from build123d import *

# Parameters (mm, degrees)
SWEEP_THIN1_PROFILE_R   = 10
SWEEP_THIN1_PROFILE_R_2 = 7
CUT_EXTRUDE1_DEPTH      = 533.134800358
CUT_EXTRUDE1_DEPTH_BACK = 533.134800358
SKETCH22_R              = 5


with BuildPart() as part:
    # Sweep-Thin1: sweep along a path in Sketch1
    with BuildLine(Plane(origin=(0, 0, 0), x_dir=(1, 0, 0), z_dir=(0, 1, 0))) as sweep_thin1_path:
        Line((0, 0), (-162.634559673, 162.634559673))
        ThreePointArc((-162.634559673, 162.634559673), (-178.855727114, 173.473197239), (-197.989898732, 177.279220614))
        Line((-197.989898732, 177.279220614), (-497.989898732, 177.279220614))
    # Sweep-Thin1 profile (on start of the path) → Sweep-Thin1 (sweep)
    with BuildSketch(Plane(origin=(0, 0, 0), x_dir=(-0.7071067811865488, 0, 0.7071067811865464), z_dir=(-0.7071067811865464, 0, -0.7071067811865488))):
        Circle(SWEEP_THIN1_PROFILE_R)
        Circle(SWEEP_THIN1_PROFILE_R_2, mode=Mode.SUBTRACT)
    sweep(path=sweep_thin1_path.line)

    # Sketch22 → Cut-Extrude1 (cut, two sides: drawn at the far end of the back side and taken through both)
    with BuildSketch(Plane(origin=(0, 0, 0), x_dir=(1, 0, 0), z_dir=(0, 1, 0)).offset(-CUT_EXTRUDE1_DEPTH_BACK)):
        with Locations(Location((-35.355339059, 35.355339059, 0), (0, 0, 270))):
            Circle(SKETCH22_R)
    extrude(amount=CUT_EXTRUDE1_DEPTH + CUT_EXTRUDE1_DEPTH_BACK, mode=Mode.SUBTRACT)


solid = part.part
Geometry check sheet. Reference: the model listing, model coordinates, mm. A direction names the side the tool comes from. Coordinates: 2 decimals unless noted, no trailing zeros. Order: outer loops, then holes, each group sorted by start corner. A loop starts at its lowest first (then second) coordinate and runs counter-clockwise, first axis right, second up. Notation, with made-up numbers: (-5.75, 71) -> (37.25, 71) arc R24 cw to (37.25, 85) -> close; hole circle Ø7 at (-30, 51.5). An arc over 180 degrees is marked (long way). Use a Markdown table: item, result. Add a question column.
1. Material ranges on L1, parallel to X at y = -1.75, z = -118; L2, parallel to Z at x = -389.5, y = 2.5; L3, parallel to Z at x = -441.5, y = -1.25, recorded low to high.
2. Set-up check for faces 1 (the face through (-350.09, 0.44, -187.27)), 2 (the face through (-87.177, 2.103, -77.735)): record each of +Z, -Z, +X, -X, +Y, -Y from which the full face is reachable in a straight line by a thin tool's end or side.
3. Mould release check, pull along Y, two halves, no side actions. Record for faces 3 (the face through (5, -2, -5)), 4 (the face through (-86.26, 8.43, -78.65)), 5 (the face through (-350.1, 2.1, -170.6)): pulls with the +Y half, pulls with the -Y half, needs draft (parallel to the pull), parting line crosses it, or undercut.
4. Go/stop test with flat-tipped pins: pin 1 Ø8 at (x, z) = (-35.36, -35.36) entering from -Y; pin 2 Ø3 at (y, z) = (7.5, -150) entering from -X; pin 3 Ø10 at (y, z) = (0, -104.5) entering from +X; pin 4 Ø12 at (x, y) = (-421.5, -3.5) entering from +Z. Record where each tip stops, or that it passes through.
5. Cross-section at A-A (x = -399). Enter the section's corners in (y, z).
6. Cross-section at B-B (y = 0). Enter the section's corners in (x, z).
Filled sheet:
| question | item | result |
|---|---|---|
| 1 | L1 | -131.92 to -127.59, -108.41 to -104.08 |
| 1 | L2 | -186.96 to -183.82, -170.74 to -167.6 |
| 1 | L3 | -187.2 to -184.17, -170.39 to -167.36 |
| 2 | face 1 | -X |
| 2 | face 2 | none |
| 3 | face 3 | needs draft |
| 3 | face 4 | parting line crosses it |
| 3 | face 5 | undercut |
| 4 | pin 1 | through |
| 4 | pin 2 | x = -161.89 |
| 4 | pin 3 | x = -85.36 |
| 4 | pin 4 | z = -167.28 |
| 5 | outline | circle Ø20 at (0, -177.28); hole circle Ø14 at (0, -177.28) |
| 6 | outline | (-497.99, -187.28) -> (-197.99, -187.28) arc R60 ccw to (-155.56, -169.71) -> (7.07, -7.07) -> (4.95, -4.95) -> (-157.68, -167.58) arc R57 cw to (-197.99, -184.28) -> (-497.99, -184.28) -> close; (-497.99, -170.28) -> (-197.99, -170.28) arc R43 ccw to (-167.58, -157.68) -> (-4.95, 4.95) -> (-7.07, 7.07) -> (-169.71, -155.56) arc R40 cw to (-197.99, -167.28) -> (-497.99, -167.28) -> close |
